Read the model definition and answer for the solid it produces. Units are mm, in the model's axes. A direction names the side the tool comes from. Coordinates: 2 decimals unless noted, no trailing zeros. Write each loop counter-clockwise with the first axis right and the second up, starting at its lowest first coordinate (ties: lowest second). Pieces come first, ordered by that corner, then holes.
Item 1: Straight lines are drawn through the part: probe 1 along X at (y, z) = (0, 26) (3 decimals); probe 2 along Z at (x, y) = (15.5, -9); probe 3 along Z at (x, y) = (16, 1). For each, find the intervals that lie inside material, in ascending order.
Item 2: Section D-D (x = 65.5) is taken. Give the vertices of the cut face in (y, z), then the cut area to 3 significant figures.
Item 3: Determine the mould class of faces 6 (the face through (17.3, -24.84, -1.78)), 7 (the face through (15.47, -0.152, -18.397)), 8 (the face through (26, -1, 68.908)), 9 (the face through (60, 35, 59)) for opening direction Z: released by +Z, released by -Z, zero draft, split by the parting line, or undercut.
Item 4: Section C-C (z = 59.5) is taken. Give the vertices of the cut face in (x, y).
Item 5: A tool of negligible diameter and unlimited length cuts with its end or side. For faces 1 (the face through (19.7, 8.73, -6.69)), 2 (the face through (3, -1, -35.591)), 3 (the face through (17.3, -1.78, 24.84)), 4 (the face through (17.14, 24.84, -1.97)), 5 (the face through (39.954, 3, -11)), from which of +Z, -Z, +X, -X, +Y, -Y can it reach the whole face along a straight path? Write none if from no direction.
Item 6: Each of these flat-tipped pins is pushed along its axis until it touches: P1, Ø6.5, axis at x = 14.986, y = 0, coming from the -Z side; P2, Ø1.5, axis at y = -16, z = -3.5, coming from the +X side; P3, Ø6.5, axis at x = 14.986, z = 0, coming from the +Y side. Where does it stop, or does it pass through?
Item 7: Section B-B (y = 44) is taken. Give the vertices of the cut face in (x, z), then the cut area to 3 significant figures.
Item 8: Section A-A (x = 31.5) is taken. Give the vertices of the cut face in (y, z), then the cut area to 3 significant figures.
from build123d import *

# Parameters (mm, degrees)
F0_R      = 29.972
F1_DEPTH  = 29.972
F2_R      = 17.9959
F3_DEPTH  = 9.9822
F5_D      = 21.9964
F6_SIZE   = 1.778
F7_SIZE   = 1.778
F14_D     = 5.842
F14_DEPTH = 9.9822
F14_START = 0.1680766
F14_TIP   = 1.7551138682
F15_D     = 5.842
F15_DEPTH = 9.9822
F15_START = 0.1680766
F15_TIP   = 1.7551138682
F18_D     = 5.842
F18_DEPTH = 9.9822
F18_START = 0.1680766
F18_TIP   = 1.7551138682
F19_D     = 5.842
F19_DEPTH = 9.9822
F19_START = 0.1680766
F19_TIP   = 1.7551138682
F20_SIZE  = 1.778
F22_DEPTH = 50
F23_SIZE  = 30
F24_SIZE  = 30


with BuildPart() as f1:
    # F0 (on Right) → F1 (new body)
    with BuildSketch(Plane.YZ):
        Circle(F0_R)
    extrude(amount=F1_DEPTH)

    # F2 (on face) → F3 (join)
    with BuildSketch(Plane.YZ.offset(29.972)):
        Circle(F2_R)
    extrude(amount=F3_DEPTH)

    # F5 (through all)
    with Locations(Plane.YZ.offset(39.9542)):
        with Locations((0, 0)):
            Hole(F5_D / 2)

    # F6
    f6_edges = [f1.edges().sort_by_distance(p)[0] for p in [
        (0, -29.972, 0),
    ]]
    chamfer(f6_edges, length=F6_SIZE)

    # F7
    f7_edges = [f1.edges().sort_by_distance(p)[0] for p in [
        (29.972, -29.972, 0),
    ]]
    chamfer(f7_edges, length=F7_SIZE)

    # F14
    # its depths count from where the whole tool has entered the part; down to there all is cleared
    with Locations(Plane(origin=(0, 29.9974, 0), x_dir=(1, 0, 0), z_dir=(0, 1, 0)).offset(-F14_START)):
        with Locations((14.986, 0)):
            Hole(F14_D / 2, depth=F14_DEPTH)
            with Locations((0, 0, -(F14_DEPTH + F14_TIP / 2))):  # 118° drill point
                Cone(0, F14_D / 2, F14_TIP, mode=Mode.SUBTRACT)

    # F15
    # its depths count from where the whole tool has entered the part; down to there all is cleared
    with Locations(Plane.XZ.offset(29.9974).offset(-F15_START)):
        with Locations((14.986, 0)):
            Hole(F15_D / 2, depth=F15_DEPTH)
            with Locations((0, 0, -(F15_DEPTH + F15_TIP / 2))):  # 118° drill point
                Cone(0, F15_D / 2, F15_TIP, mode=Mode.SUBTRACT)

    # F18
    # its depths count from where the whole tool has entered the part; down to there all is cleared
    with Locations(Plane(origin=(0, 0, -29.9974), x_dir=(1, 0, 0), z_dir=(0, 0, -1)).offset(-F18_START)):
        with Locations((14.986, 0)):
            Hole(F18_D / 2, depth=F18_DEPTH)
            with Locations((0, 0, -(F18_DEPTH + F18_TIP / 2))):  # 118° drill point
                Cone(0, F18_D / 2, F18_TIP, mode=Mode.SUBTRACT)

    # F19
    # its depths count from where the whole tool has entered the part; down to there all is cleared
    with Locations(Plane.XY.offset(29.9974).offset(-F19_START)):
        with Locations((14.986, 0)):
            Hole(F19_D / 2, depth=F19_DEPTH)
            with Locations((0, 0, -(F19_DEPTH + F19_TIP / 2))):  # 118° drill point
                Cone(0, F19_D / 2, F19_TIP, mode=Mode.SUBTRACT)

    # F20
    f20_edges = [f1.edges().sort_by_distance(p)[0] for p in [
        (39.9542, -17.9959, 0),
    ]]
    chamfer(f20_edges, length=F20_SIZE)

    # F21 (on Front) → F22 (join, symmetric)
    with BuildSketch(Plane.XZ):
        Polygon((-25, -45), (0, -45), (4.9744802527, -45), (4.9744802527, -35.5912335217), (0, -35.5912335217), (0, 0), (0, 48.9084279899), (75, 48.9084279899), (75, 68.9084279899), (-25, 68.9084279899), align=None)
    extrude(amount=F22_DEPTH, both=True)

    # F23
    f23_edges = [f1.edges().sort_by_distance(p)[0] for p in [
        (75, -50, 58.908428),
    ]]
    chamfer(f23_edges, length=F23_SIZE)

    # F24
    f24_edges = [f1.edges().sort_by_distance(p)[0] for p in [
        (75, 50, 58.908428),
    ]]
    chamfer(f24_edges, length=F24_SIZE)


solid = f1.part
Established:
1. probe 1: x = -25 to 12.065, 17.907 to 29.972
1. probe 2: z = -28.59 to -6.32, 6.32 to 28.59, 48.91 to 68.91
1. probe 3: z = -18.95 to -10.95, 10.95 to 18.95, 48.91 to 68.91
2. outline: (-29.5, 48.91) - (29.5, 48.91) - (29.5, 68.91) - (-29.5, 68.91) - close
2. area: 1,180 mm2
3. face 6: undercut
3. face 7: released by -Z
3. face 8: released by +Z
3. face 9: zero draft
4. outline: (-25, -50) - (45, -50) - (75, -20) - (75, 20) - (45, 50) - (-25, 50) - close
5. face 1: +X
5. face 2: +X, +Y, -Y
5. face 3: none
5. face 4: +Y
5. face 5: -Z, +X, +Y, -Y
6. P1: stops at z = -29.97
6. P2: stops at x = 39.95
6. P3: stops at y = 29.97
7. outline: (-25, -45) - (4.97, -45) - (4.97, -35.59) - (0, -35.59) - (0, 48.91) - (51, 48.91) - (51, 68.91) - (-25, 68.91) - close
7. area: 3,910 mm2
8. outline: (-50, 48.91) - (50, 48.91) - (50, 68.91) - (-50, 68.91) - close; circle Ø35.99 at (0, 0); hole circle Ø22 at (0, 0)
8. area: 2,640 mm2
